Autodesk Inventor part; units mm, degrees
ref_plane "YZ Plane" through (0, 0, 0) normal (1, 0, 0) x (0, 1, 0)
ref_plane "XZ Plane" through (0, 0, 0) normal (0, 1, 0) x (-1, 0, 0)
ref_plane "XY Plane" through (0, 0, 0) normal (0, 0, 1) x (1, 0, 0)
ref_plane "Work Plane5" through (0, 3, 0) normal (0, 1, 0) x (1, 0, 0)
sketch "Sketch45" plane through (0, 3, 0) normal (0, 1, 0) x (1, 0, 0)
  line L0 (35, -20) -> (-3, -20)
  line L1 (-3, -20) -> (-3, 20)
  line L2 (-3, 20) -> (35, 20)
  line L3 (35, 20) -> (35, -20)
  point P0 (0, 0)
  dimension "d142" = 38
  dimension "d143" = 40
extrude "Extrusion34" add sketch "Sketch45" along normal blind 30
ref_plane "Work Plane2" through (0, 0, 0) normal (0, -1, 0) x (1, 0, 0)
sketch "Sketch47" plane through (0, 0, 0) normal (0, -1, 0) x (1, 0, 0)
  circle A0 centre (16, 0) radius 18
  point P0 (0, 0)
  dimension "d146" = 36
extrude "Extrusion35" cut sketch "Sketch47" against normal blind 30 draft -15
ref_plane "Work Plane1" through (0, 3, 0) normal (0, 1, 0) x (1, 0, 0)
sketch "Sketch74" plane through (0, 33, 0) normal (0, 1, 0) x (1, 0, 0)
  circle A0 centre (20, 0) radius 1.15
  point P0 (0, 0)
  dimension "d210" = 2.3
extrude "Extrusion51" cut sketch "Sketch74" against normal blind 10
sketch "Sketch77" plane through (0, 3, 0) normal (0, -1, 0) x (1, 0, 0)
  circle A0 centre (16, 0) radius 17.5
  point P0 (0, 0)
  dimension "d219" = 35
sketch "Sketch78" plane through (0, 3, 0) normal (0, -1, 0) x (1, 0, 0)
  line L0 (45, -30) -> (-13, -30)
  line L1 (-13, -30) -> (-13, 30)
  line L2 (-13, 30) -> (45, 30)
  line L3 (45, 30) -> (45, -30)
  line L4 (45, -30) -> (-13, 30) construction
  line L5 (-13, -30) -> (45, 30) construction
  point P0 (0, 0)
  point P1 (16, 0)
  dimension "d220" = 58
  dimension "d221" = 60
extrude "Extrusion53" add sketch "Sketch78" against normal blind 3
extrude "Extrusion54" cut sketch "Sketch77" against normal blind 3
sketch "Sketch79" plane through (0, 6, 0) normal (0, 1, 0) x (1, 0, 0)
  circle A0 centre (16, -25) radius 3.35
  circle A1 centre (16, 25) radius 3.35
  circle A2 centre (40, 0) radius 3.35
  point P0 (0, 0)
  dimension "d226" = 6.7
  dimension "d227" = 6.7
  dimension "d228" = 6.7
extrude "Extrusion55" cut sketch "Sketch79" against normal through all
properties part number "liquid_port_v01"
Model file for the job. Use its own axes, mm. A direction names the side the tool comes from. Round coordinates to 2 decimals unless told otherwise and drop trailing zeros. Loops run counter-clockwise (first coordinate to the right, second up) from the corner with the lowest first, then second, coordinate; pieces in that order, holes last. Notation, with made-up numbers: M -2,41 L 46,41 A5 cw 46,49 Z; hole C 84.5,-24 d7. An arc over 180 degrees is marked long. Put each result on its own line as item: value. Start each with the question number.
Item 1: Drill centre lines: line 1 along Z through (x, y) = (16, 5.3); line 2 along Z through (x, y) = (40, 4.5); line 3 along Z through (x, y) = (28, 30). Where is each one in solid material? Low to high.
Item 2: Drop flat-ended pins along their axis: P1, Ø8, axis at y = 21.5, z = -5.5, coming from the +X side; P2, Ø4, axis at y = 15.5, z = -21.5, coming from the -X side; P3, Ø10.5, axis at x = 16, z = 25, coming from the +Y side; P4, Ø8.5, axis at x = 16, z = -25, coming from the +Y side. Give the stop position or say it passes through.
Item 3: Cut at C-C (z = -25). List the corners of the cut face in (x, y), then the cut area to 3 significant figures.
Item 4: Cut at D-D (x = 40). List the corners of the cut face in (y, z).
Item 5: 3-axis set-ups, long thin cutter, end or side, ignore diameter. For faces 1 (the face through (2.113, 4.479, -10.648)), 2 (the face through (16, 19, -20)), 3 (the face through (-3, 19, 0)): which of +Z, -Z, +X, -X, +Y, -Y reach the whole face in a straight line?
Item 6: Cut at A-A (z = 0). List the corners of the cut face in (x, y).
Item 7: Cut at B-B (x = 16). List the corners of the cut face in (y, z), then the cut area to 3 significant figures.
Item 8: Mould opens along X. For faces 4 (the face through (16, 30, 0)), 5 (the face through (35, 19, 0)), 6 (the face through (3, 3, 14)), 7 (the face through (18.85, 31.52, -0.05)) say: released by +X, released by -X, zero draft, split by the parting line, or undercut.
Answer block:
1. line 1: -30 to -28.35, -21.65 to -17.5, 17.5 to 21.65, 28.35 to 30
1. line 2: -30 to -3.35, 3.35 to 30
1. line 3: -20 to 20
2. P1: x = 35
2. P2: x = -3
2. P3: y = 33
2. P4: y = 6
3. outline: M -13,3 L 12.65,3 L 12.65,6 L -13,6 Z; M 19.35,3 L 45,3 L 45,6 L 19.35,6 Z
3. area: 154 mm2
4. outline: M 3,-30 L 6,-30 L 6,-3.35 L 3,-3.35 Z; M 3,3.35 L 6,3.35 L 6,30 L 3,30 Z
5. face 1: -Y
5. face 2: -Z, +X, -X, +Y
5. face 3: +Z, -Z, -X, +Y
6. outline: M -13,3 L -1.5,3 L -1.5,6 L -0.39,6 L 6.04,30 L 18.85,30 L 18.85,33 L -3,33 L -3,6 L -13,6 Z; M 21.15,30 L 25.96,30 L 32.39,6 L 33.5,6 L 33.5,3 L 36.65,3 L 36.65,6 L 35,6 L 35,33 L 21.15,33 Z; M 43.35,3 L 45,3 L 45,6 L 43.35,6 Z
7. outline: M 3,-30 L 6,-30 L 6,-28.35 L 3,-28.35 Z; M 3,-21.65 L 6,-21.65 L 6,-20 L 33,-20 L 33,20 L 6,20 L 6,21.65 L 3,21.65 L 3,17.5 L 6,17.5 L 6,16.39 L 30,9.96 L 30,-9.96 L 6,-16.39 L 6,-17.5 L 3,-17.5 Z; M 3,28.35 L 6,28.35 L 6,30 L 3,30 Z
7. area: 482 mm2
8. face 4: undercut
8. face 5: released by +X
8. face 6: zero draft
8. face 7: undercut
